Verification items for the finished model (mm, model axes). A direction names the side the tool comes from. Give positions to 0.01 mm unless a question says otherwise; leave off trailing zeros. Loops run counter-clockwise (first coordinate to the right, second up) from the corner with the lowest first, then second, coordinate; pieces in that order, holes last. Notation, with made-up numbers: (-2, -36.5) - (47, -36.5) arc R8 cw to (47, -24.5) - close; hole circle Ø11 at (62.25, -11). An arc over 180 degrees is marked (long way). One line per item, written item: value. Start each with the question number.
1. Sectioned sample at A-A (y = -1.5). Record the cut outline in (x, z), plus the area to 3 significant figures.
2. Scan lines: L1, parallel to Y at x = 24.5, z = 0.25; L2, parallel to X at y = -5, z = 0.3; L3, parallel to Y at x = -1.5, z = 1.45. Record each from-to range of solid material in increasing order. Write a range as [from, to].
3. Sectioned sample at B-B (z = 1). Count the separate pieces of the cut face and the enclosed holes in it, plus the area to 3 significant figures.
4. Access from +Z, -Z, +X, -X, +Y, -Y to the whole of each face (thin tool, end or side, straight path). Record for faces 5 (the cylindrical face through (-35.3, -17.5, 0.7)), 6 (the cylindrical face through (39.4, -21.98, 0.74)), 7 (the cylindrical face through (-17.5, 35.3, 0.7)).
5. Mould release check, pull along Y, two halves, no side actions. Record for faces 1 (the cylindrical face through (-16.43, -14.17, 0.74)), 2 (the cylindrical face through (-21.98, -39.4, 0.74)), 3 (the flat face through (33.364, 33.153, 0.74)), 4 (the flat face through (7.63, 0.95, 0.74)): pulls with the +Y half, pulls with the -Y half, needs draft (parallel to the pull), parting line crosses it, or undercut.
6. Gauge pin test, flat ends, axial feed: pin 1 (10 mm diameter, centred on x = 4, y = -0.5, fed in from -Z); pin 2 (3 mm diameter, centred on x = -15.25, y = -15.25, fed in from +Z); pin 3 (0.8 mm diameter, centred on x = -1, z = 1, fed in from -Y). Record the tip position at first contact, or that the pin passes through.
from build123d import *

# Parameters (mm, degrees)
F0_R     = 2.225
F0_R_2   = 1.6
F0_R_3   = 2.25
F1_DEPTH = 1.5


# Not quite as in the source:
# - ends of sketch curves that miss each other by under 0.0002 mm in the source are joined


with BuildPart() as f1:
    # F0 (on Top) → F1 (new body)
    with BuildSketch(Plane.XY):
        with BuildLine():
            Line((40.764131, 25.752812), (25.752812, 40.764131))
            ThreePointArc((25.752812, 40.764131), (24.7844707903, 41.2006273849), (23.7698381424, 40.8864068174))
            ThreePointArc((23.7698381424, 40.8864068174), (21.9550704325, 39.3793732762), (20.2364945752, 37.7635054248))
            ThreePointArc((20.2364945752, 37.7635054248), (17.5612326137, 35.3520830837), (14.6508446305, 33.2303795663))
            ThreePointArc((14.6508446305, 33.2303795663), (8.9914965544, 30.4470141229), (2.8299590067, 29.1013549294))
            ThreePointArc((2.8299590067, 29.1013549294), (0, 28.968262), (-2.8299590155, 29.1013548358))
            ThreePointArc((-2.8299590155, 29.1013548358), (-8.9914965544, 30.4470141229), (-14.6508445509, 33.2303796882))
            ThreePointArc((-14.6508445509, 33.2303796882), (-17.5612326137, 35.3520830837), (-20.2364941171, 37.7635058829))
            ThreePointArc((-20.2364941171, 37.7635058829), (-21.9550704325, 39.3793732762), (-23.7698383319, 40.8864065743))
            ThreePointArc((-23.7698383319, 40.8864065743), (-24.7844707903, 41.2006273849), (-25.7528121718, 40.7641311718))
            Line((-25.7528121718, 40.7641311718), (-40.764131, 25.752812))
            ThreePointArc((-40.764131, 25.752812), (-41.2006273849, 24.7844707903), (-40.8864068174, 23.7698381424))
            ThreePointArc((-40.8864068174, 23.7698381424), (-39.3793732762, 21.9550704325), (-37.7635054248, 20.2364945752))
            ThreePointArc((-37.7635054248, 20.2364945752), (-35.3520832558, 17.5612328258), (-33.2303798649, 14.6508450882))
            ThreePointArc((-33.2303798649, 14.6508450882), (-30.4470115556, 8.9914892045), (-29.1013534168, 2.8299429607))
            ThreePointArc((-29.1013534168, 2.8299429607), (-28.968262, 0), (-29.1013532045, -2.8299429807))
            ThreePointArc((-29.1013532045, -2.8299429807), (-30.4470115556, -8.9914892045), (-33.2303799868, -14.6508450086))
            ThreePointArc((-33.2303799868, -14.6508450086), (-35.3520832558, -17.5612328258), (-37.7635058829, -20.2364941171))
            ThreePointArc((-37.7635058829, -20.2364941171), (-39.3793732762, -21.9550704325), (-40.8864065743, -23.7698383319))
            ThreePointArc((-40.8864065743, -23.7698383319), (-41.2006273849, -24.7844707903), (-40.7641311718, -25.7528121718))
            Line((-40.7641311718, -25.7528121718), (-25.752812, -40.764131))
            ThreePointArc((-25.752812, -40.764131), (-24.7844707903, -41.2006273849), (-23.7698381424, -40.8864068174))
            ThreePointArc((-23.7698381424, -40.8864068174), (-21.9550704325, -39.3793732762), (-20.2364945752, -37.7635054248))
            ThreePointArc((-20.2364945752, -37.7635054248), (-17.5612326137, -35.3520830837), (-14.6508446305, -33.2303795663))
            ThreePointArc((-14.6508446305, -33.2303795663), (-8.9914965544, -30.4470141229), (-2.8299590067, -29.1013549294))
            ThreePointArc((-2.8299590067, -29.1013549294), (0, -28.968262), (2.8299590155, -29.1013548358))
            ThreePointArc((2.8299590155, -29.1013548358), (8.9914965544, -30.4470141229), (14.6508445509, -33.2303796882))
            ThreePointArc((14.6508445509, -33.2303796882), (17.5612326137, -35.3520830837), (20.2364941171, -37.7635058829))
            ThreePointArc((20.2364941171, -37.7635058829), (21.9550704325, -39.3793732762), (23.7698383319, -40.8864065743))
            ThreePointArc((23.7698383319, -40.8864065743), (24.7844707903, -41.2006273849), (25.7528121718, -40.7641311718))
            Line((25.7528121718, -40.7641311718), (40.764131, -25.752812))
            ThreePointArc((40.764131, -25.752812), (41.2006273849, -24.7844707903), (40.8864068174, -23.7698381424))
            ThreePointArc((40.8864068174, -23.7698381424), (39.3793732762, -21.9550704325), (37.7635054248, -20.2364945752))
            ThreePointArc((37.7635054248, -20.2364945752), (35.3520832558, -17.5612328258), (33.2303798649, -14.6508450882))
            ThreePointArc((33.2303798649, -14.6508450882), (30.4470115556, -8.9914892045), (29.1013534168, -2.8299429607))
            ThreePointArc((29.1013534168, -2.8299429607), (28.968262, 0), (29.1013532045, 2.8299429807))
            ThreePointArc((29.1013532045, 2.8299429807), (30.4470115556, 8.9914892045), (33.2303799868, 14.6508450086))
            ThreePointArc((33.2303799868, 14.6508450086), (35.3520832558, 17.5612328258), (37.7635058829, 20.2364941171))
            ThreePointArc((37.7635058829, 20.2364941171), (39.3793732762, 21.9550704325), (40.8864065743, 23.7698383319))
            ThreePointArc((40.8864065743, 23.7698383319), (41.2006273849, 24.7844707903), (40.764131, 25.752812))
        make_face()
        with Locations((-29, -29)):
            Circle(F0_R, mode=Mode.SUBTRACT)
        with Locations((-10.282726, -24.824696)):
            Circle(F0_R, mode=Mode.SUBTRACT)
        with Locations((-24.824696, -10.282726)):
            Circle(F0_R, mode=Mode.SUBTRACT)
        with Locations((-15.25, -15.25)):
            Circle(F0_R_2, mode=Mode.SUBTRACT)
        with Locations((10.282726, -24.824696)):
            Circle(F0_R, mode=Mode.SUBTRACT)
        with Locations((29, -29)):
            Circle(F0_R, mode=Mode.SUBTRACT)
        with BuildLine():
            Line((-10, -14.25), (10, -14.25))
            ThreePointArc((10, -14.25), (11, -15.25), (10, -16.25))
            Line((10, -16.25), (-10, -16.25))
            ThreePointArc((-10, -16.25), (-11, -15.25), (-10, -14.25))
        make_face(mode=Mode.SUBTRACT)
        with Locations((15.25, -15.25)):
            Circle(F0_R_2, mode=Mode.SUBTRACT)
        with Locations((24.824696, -10.282726)):
            Circle(F0_R_3, mode=Mode.SUBTRACT)
        with Locations((-24.824696, 10.282726)):
            Circle(F0_R, mode=Mode.SUBTRACT)
        with BuildLine():
            ThreePointArc((-16.25, 10), (-15.25, 11), (-14.25, 10))
            Line((-14.25, 10), (-14.25, -10))
            ThreePointArc((-14.25, -10), (-15.25, -11), (-16.25, -10))
            Line((-16.25, -10), (-16.25, 10))
        make_face(mode=Mode.SUBTRACT)
        with BuildLine():
            ThreePointArc((-0.4956958589, 0.885209945), (-0.771266673, 0.5382796173), (-1.194556, 0.407413))
            Line((-1.194556, 0.407413), (-5.541795, 0.407413))
            Line((-5.541795, 0.407413), (-8.150595, -6.290485))
            ThreePointArc((-8.150595, -6.290485), (-8.426165673, -6.6374153827), (-8.849455, -6.768282))
            Line((-8.849455, -6.768282), (-9.669691, -6.768282))
            ThreePointArc((-9.669691, -6.768282), (-10.2888243827, -6.441571327), (-10.3685511411, -5.746078945))
            Line((-10.3685511411, -5.746078945), (-4.809405, 8.526614))
            ThreePointArc((-4.809405, 8.526614), (-4.533834327, 8.8735443827), (-4.110545, 9.004411))
            Line((-4.110545, 9.004411), (4.809691, 9.004411))
            ThreePointArc((4.809691, 9.004411), (5.4288241198, 8.6777007117), (5.5085514793, 7.9822088133))
            Line((5.5085514793, 7.9822088133), (5.23237, 7.273132))
            ThreePointArc((5.23237, 7.273132), (4.9567984768, 6.9262017197), (4.533509, 6.795335))
            Line((4.533509, 6.795335), (-3.05373, 6.795335))
            Line((-3.05373, 6.795335), (-4.681371, 2.61649))
            Line((-4.681371, 2.61649), (-0.918374, 2.61649))
            ThreePointArc((-0.918374, 2.61649), (-0.2992406173, 2.289779327), (-0.2195138589, 1.594286945))
            Line((-0.2195138589, 1.594286945), (-0.4956958589, 0.885209945))
        make_face(mode=Mode.SUBTRACT)
        with Locations((-15.25, 15.25)):
            Circle(F0_R_2, mode=Mode.SUBTRACT)
        with Locations((-29, 29)):
            Circle(F0_R, mode=Mode.SUBTRACT)
        with Locations((-10.282726, 24.824696)):
            Circle(F0_R, mode=Mode.SUBTRACT)
        with BuildLine():
            ThreePointArc((3.290309, -6.768282), (2.6711756173, -6.441571327), (2.5914488589, -5.746078945))
            Line((2.5914488589, -5.746078945), (7.47627, 6.795335))
            Line((7.47627, 6.795335), (6.953273, 6.795335))
            ThreePointArc((6.953273, 6.795335), (6.3341396173, 7.122045673), (6.2544128589, 7.817538055))
            Line((6.2544128589, 7.817538055), (6.530595, 8.526614))
            ThreePointArc((6.530595, 8.526614), (6.806165673, 8.8735443827), (7.229455, 9.004411))
            Line((7.229455, 9.004411), (9.669691, 9.004411))
            ThreePointArc((9.669691, 9.004411), (10.2888241198, 8.6777007117), (10.3685514793, 7.9822088133))
            Line((10.3685514793, 7.9822088133), (4.809405, -6.290485))
            ThreePointArc((4.809405, -6.290485), (4.533834327, -6.6374153827), (4.110545, -6.768282))
            Line((4.110545, -6.768282), (3.290309, -6.768282))
        make_face(mode=Mode.SUBTRACT)
        with BuildLine():
            Line((14.25, -10), (14.25, 10))
            ThreePointArc((14.25, 10), (15.25, 11), (16.25, 10))
            Line((16.25, 10), (16.25, -10))
            ThreePointArc((16.25, -10), (15.25, -11), (14.25, -10))
        make_face(mode=Mode.SUBTRACT)
        with BuildLine():
            ThreePointArc((10, 16.25), (11, 15.25), (10, 14.25))
            Line((10, 14.25), (-10, 14.25))
            ThreePointArc((-10, 14.25), (-11, 15.25), (-10, 16.25))
            Line((-10, 16.25), (10, 16.25))
        make_face(mode=Mode.SUBTRACT)
        with Locations((15.25, 15.25)):
            Circle(F0_R_2, mode=Mode.SUBTRACT)
        with Locations((24.824696, 10.282726)):
            Circle(F0_R, mode=Mode.SUBTRACT)
        with Locations((10.282726, 24.824696)):
            Circle(F0_R, mode=Mode.SUBTRACT)
        with Locations((29, 29)):
            Circle(F0_R, mode=Mode.SUBTRACT)
    extrude(amount=F1_DEPTH)


solid = f1.part
Results are:
1. outline: (-29.01, 0) - (-16.25, 0) - (-16.25, 1.5) - (-29.01, 1.5) - close; (-14.25, 0) - (-8.71, 0) - (-8.71, 1.5) - (-14.25, 1.5) - close; (-6.28, 0) - (4.25, 0) - (4.25, 1.5) - (-6.28, 1.5) - close; (6.68, 0) - (14.25, 0) - (14.25, 1.5) - (6.68, 1.5) - close; (16.25, 0) - (29.01, 0) - (29.01, 1.5) - (16.25, 1.5) - close
1. area: 73.7 mm^2
2. L1: y = [-41.19, -12.51], [-8.06, 8.08], [12.48, 41.19]
2. L2: x = [-29.4, -16.25], [-14.25, -10.08], [-7.65, 2.88], [5.31, 14.25], [16.25, 29.4]
2. L3: y = [-29.01, -16.25], [-14.25, 0.41], [2.62, 6.8], [9, 14.25], [16.25, 29.01]
3. separate pieces: 1
3. enclosed holes: 22
3. area: 4,200 mm^2
4. face 5: +Z, -Z, -X
4. face 6: +Z, -Z, +X
4. face 7: +Z, -Z, +Y
5. face 1: undercut
5. face 2: pulls with the -Y half
5. face 3: pulls with the +Y half
5. face 4: undercut
6. pin 1: stops at z = 0
6. pin 2: passes through
6. pin 3: stops at y = -29
